Can you work these out from the model? Positions are in its coordinate system, mm. A direction names the side the tool comes from. Coordinates: 2 decimals unless noted, no trailing zeros. Order: outer loops, then holes, each group sorted by start corner. A loop starts at its lowest first (then second) coordinate and runs counter-clockwise, first axis right, second up. Notation, with made-up numbers: (33, -39) -> (75, -39) arc R20 ccw to (75, -20) -> close; hole circle Ø5 at (56, -37.75). An arc over 180 degrees is marked (long way). Answer as a JSON object with one key per item and string values. Group by question number.
(1) Which directions (+Z, -Z, +X, -X, +Y, -Y) give clear straight access to the entire face, cutting with the end or side of a thin tool? Please do faces 1 (the flat face through (-8.489, 7, 7)), 2 (the flat face through (15, 3.605, 7)), 3 (the flat face through (0, -2.745, 7)).
(2) I need wall thicknesses on line 1 (Y direction, x = -14, z = 0.75); line 2 (X direction, y = 6.75, z = 2); line 3 (X direction, y = 8, z = 3.75). Which ranges of each line are inside material? Lowest first, please.
(3) For pin 1 (5 mm diameter, centred on y = 8, z = 7.5, fed in from -X); pin 2 (5 mm diameter, centred on x = -12.5, z = 5.5, fed in from +Y); pin 3 (1.5 mm diameter, centred on x = 0.5, z = 13, fed in from +Y), each with a flat end and sliding along its axis, tell me the tip position at first contact or that it passes through.
(4) I want a section at D-D, the plane x = -12. List the corners of the cut face in (y, z) for me, plus the area to 3 significant figures.
(5) If we mould it in two halves opening along X, with no side actions, what happens to faces 4 (the flat face through (10.815, 7, 7)), 5 (the cylindrical face through (0.667, 2.882, 7.469)), 6 (the flat face through (9, 9.955, 7))? For each: pulls with the +X half, pulls with the -X half, needs draft (parallel to the pull), parting line crosses it, or undercut.
(6) I want a section at A-A, the plane y = 4.25. List the corners of the cut face in (x, z) for me.
(7) I want a section at C-C, the plane y = 6.5. List the corners of the cut face in (x, z) for me, plus the area to 3 significant figures.
from build123d import *

# Parameters (mm, degrees)
F1_W     = 19.304
F1_H     = 6.35
F2_DEPTH = 14.732
F0_W     = 38.1
F0_H     = 6.35
F3_DEPTH = 14.732
F5_R     = 7.186013
F6_DEPTH = 14.733


with BuildPart() as f2:
    # F1 (on face) → F2 (new body)
    with BuildSketch(Plane.XY):
        with Locations((1.162567, 6.780102)):
            Rectangle(F1_W, F1_H)
    extrude(amount=F2_DEPTH)

    # F0 (on Top) → F3 (join)
    with BuildSketch(Plane.XY):
        with Locations((0.559317, 0.430102)):
            Rectangle(F0_W, F0_H)
    extrude(amount=F3_DEPTH)

    # F5 (on face) → F6 (cut, through all)
    with BuildSketch(Plane.XY.offset(14.732)):
        with Locations((0.823092, 10.066757)):
            Circle(F5_R)
    extrude(amount=-F6_DEPTH, mode=Mode.SUBTRACT)


solid = f2.part
Computed values:
{
 "1": {"face 1": "+Z, -Z, -X, +Y", "face 2": "+Z, -Z, +X, +Y", "face 3": "+Z, -Z, +X, -X, -Y"},
 "2": {"line 1": "y = -2.74 to 3.61", "line 2": "x = -8.49 to -5.55, 7.2 to 10.81", "line 3": "x = -8.49 to -6.06, 7.71 to 10.81"},
 "3": {"pin 1": "stops at x = -8.49", "pin 2": "stops at y = 3.61", "pin 3": "stops at y = 2.96"},
 "4": {"outline": "(-2.74, 0) -> (3.61, 0) -> (3.61, 14.73) -> (-2.74, 14.73) -> close", "area": "93.5 mm2"},
 "5": {"face 4": "pulls with the +X half", "face 5": "undercut", "face 6": "needs draft"},
 "6": {"outline": "(-8.49, 0) -> (-3.4, 0) -> (-3.4, 14.73) -> (-8.49, 14.73) -> close; (5.04, 0) -> (10.81, 0) -> (10.81, 14.73) -> (5.04, 14.73) -> close"},
 "7": {"outline": "(-8.49, 0) -> (-5.42, 0) -> (-5.42, 14.73) -> (-8.49, 14.73) -> close; (7.06, 0) -> (10.81, 0) -> (10.81, 14.73) -> (7.06, 14.73) -> close", "area": "101 mm2"}
}
